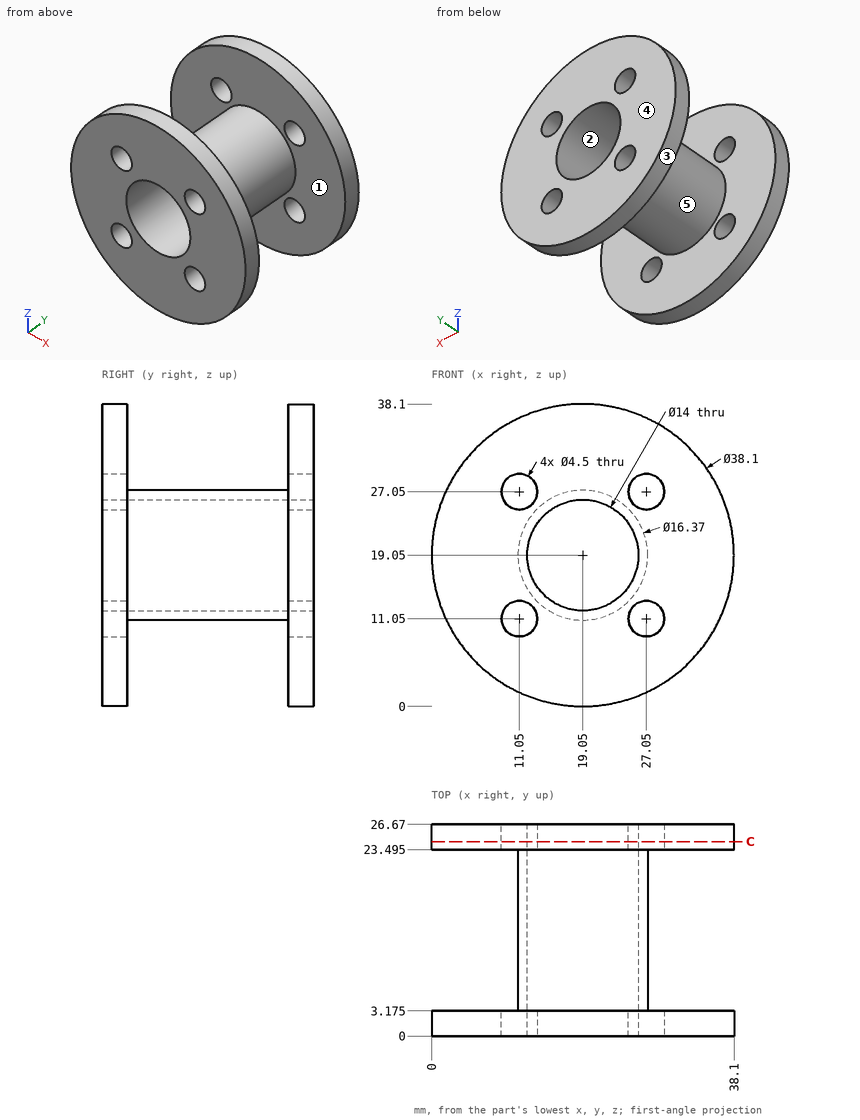
Verification items for this drawing (mm, ordinates from the low corner). A direction names the side the tool comes from. Give positions to 0.01 mm unless a question says otherwise; leave off trailing zeros. Write each loop counter-clockwise with the first axis right and the second up, starting at its lowest first coordinate (ties: lowest second). Pieces come first, ordered by that corner, then holes. Notation, with made-up numbers: (78, 17.25) -> (85, 17.25) arc R30 ccw to (85, 56.25) -> close; hole circle Ø11 at (5, 37.25). An arc over 180 degrees is marked (long way). Use CSV: the item, a comma, the result in double quotes. Start each with the question number.
Q1. Release check for a two-part mould opening along Y. For the marked faces 3, 4 and 5 record: +Y half, -Y half, draft (parallel to the pull), parting line (faces both ways), or undercut.
Q2. Tool access check on the marked faces 1 and 2. Record the directions out of +Z, -Z, +X, -X, +Y, -Y that give a thin tool (end or side, any length) a straight path to the whole face; none if there is none.
Q3. Depth check by flat-ended pin: P1, Ø10, axis at x = 23.5, y = 11, coming from the -Z side (1 decimal); P2, Ø1.5, axis at y = 14.5, z = 15, coming from the +X side; P3, Ø12, axis at y = 8, z = 32.5, coming from the +X side (1 decimal). Enter the tip coordinate at first touch or a pass-through.
Q4. Cross-section at C-C on y = 24.5. Enter the section's corners in (x, z).
Q5. Scan lines: line 1 along Y through (x, z) = (7, 31) (1 decimal); line 2 along Z through (x, y) = (11.05, 25.85). Record each from-to range of solid material in increasing order.
Working result:
1,face 3,"draft"
1,face 4,"+Y half"
1,face 5,"undercut"
2,face 1,"none"
2,face 2,"+Y, -Y"
3,P1,"stops at z = 10.9"
3,P2,"stops at x = 26.54"
3,P3,"stops at x = 35.3"
4,outline,"circle Ø38.1 at (19.05, 19.05); hole circle Ø4.5 at (11.05, 11.05); hole circle Ø4.5 at (11.05, 27.05); hole circle Ø14 at (19.05, 19.05); hole circle Ø4.5 at (27.05, 11.05); hole circle Ø4.5 at (27.05, 27.05)"
5,line 1,"y = 0 to 3.2, 23.5 to 26.7"
5,line 2,"z = 1.76 to 8.8, 13.3 to 24.8, 29.3 to 36.34"
